Source: CAD feature listing. Evaluate the final solid. Frame: model axes, mm. A direction names the side the tool comes from. Round coordinates to 2 decimals unless told otherwise and drop trailing zeros. Order: outer loops, then holes, each group sorted by start corner. A loop starts at its lowest first (then second) coordinate and runs counter-clockwise, first axis right, second up. Notation, with made-up numbers: (-28.5, 2.5) -> (16.5, 2.5) arc R7 ccw to (16.5, 9.5) -> close; hole circle Ø6 at (78.5, 54.25). An arc over 180 degrees is marked (long way). Answer as CSV lines item,"result". Start each with the question number.
(1) Section query B-B (y = -12.5). Output: boundary loops of the cut face in (x, z).
(2) Set-up query: faces 5 (the flat face through (52, -12, 10)), 6 (the flat face through (75, -12, 2)), 7 (the flat face through (-52, -12, 10)). Return all of +Z, -Z, +X, -X, +Y, -Y with unobstructed straight access to the full face (end or side cutting, diameter ignored); none if empty.
(3) Contact query for flat-ended pins moving along their axis: P1, Ø12, axis at y = -13.5, z = 44, coming from the -X side; P2, Ø2, axis at y = -6.5, z = 26.5, coming from the -X side; P3, Ø10, axis at x = 52, y = -10, coming from the +Z side; P4, Ø13.5, axis at x = 60, y = -12.5, coming from the +Z side. Output: stop coordinate, or through.
(4) Pull-direction query (Y, two-part tool) for faces 1 (the flat face through (-1, -25, 22)), 2 (the cylindrical face through (52.507, -12.17, 5.07)), 3 (the cylindrical face through (-67.493, -12.17, 5.07)), 4 (the flat face through (-1, -12, 0)); classes: +Y half, -Y half, draft (parallel to the pull), parting line (faces both ways), or undercut.
(5) Line query: line 1 along X through (y, z) = (-9.75, 8); line 2 along Y through (x, z) = (60, 6); line 3 along Z through (x, y) = (-57.5, -2.5). Output: solid intervals per line, ascending. Write a range as from..to.
(6) Section query A-A (x = 60). Output: boundary loops of the cut face in (y, z), plus the area to 3 significant figures.
(7) Section query D-D (x = -54.5). Output: boundary loops of the cut face in (y, z), plus the area to 3 significant figures.
(8) Section query C-C (y = -22.25). Output: boundary loops of the cut face in (x, z).
```python
from build123d import *

# Parameters (mm, degrees)
F1_DEPTH = 25
F2_R     = 7.5
F3_DEPTH = 10.001


with BuildPart() as f1:
    # F0 (on Front) → F1 (new body)
    with BuildSketch(Plane.XZ):
        with BuildLine():
            Line((-45, 10), (-45, 0))
            Line((-45, 0), (45, 0))
            Line((45, 0), (45, 10))
            ThreePointArc((45, 10), (31.819805, 41.819805), (0, 55))
            ThreePointArc((0, 55), (-31.819805, 41.819805), (-45, 10))
        make_face()
        with BuildLine():
            Line((-75, 5), (-75, 0))
            Line((-75, 0), (-45, 0))
            Line((-45, 0), (-45, 10))
            Line((-45, 10), (-70, 10))
            ThreePointArc((-70, 10), (-73.535534, 8.535534), (-75, 5))
        make_face()
        with BuildLine():
            Line((45, 10), (45, 0))
            Line((45, 0), (75, 0))
            Line((75, 0), (75, 5))
            ThreePointArc((75, 5), (73.535534, 8.535534), (70, 10))
            Line((70, 10), (45, 10))
        make_face()
    extrude(amount=F1_DEPTH)

    # F2 (on face) → F3 (cut, through all)
    with BuildSketch(Plane.XY.offset(10)):
        with Locations((-60, -12.5)):
            Circle(F2_R)
        with Locations((60, -12.5)):
            Circle(F2_R)
    extrude(amount=-F3_DEPTH, mode=Mode.SUBTRACT)


solid = f1.part
```
Answer block:
1,outline,"(-75, 0) -> (-67.5, 0) -> (-67.5, 10) -> (-70, 10) arc R5 ccw to (-75, 5) -> close; (-52.5, 0) -> (52.5, 0) -> (52.5, 10) -> (45, 10) arc R45 ccw to (0, 55) arc R45 ccw to (-45, 10) -> (-52.5, 10) -> close; (67.5, 0) -> (75, 0) -> (75, 5) arc R5 ccw to (70, 10) -> (67.5, 10) -> close"
2,face 5,"+Z, +X, +Y, -Y"
2,face 6,"+Z, -Z, +X, +Y, -Y"
2,face 7,"+Z, -X, +Y, -Y"
3,P1,"x = -35.23"
3,P2,"x = -42.25"
3,P3,"z = 10"
3,P4,"through"
4,face 1,"-Y half"
4,face 2,"undercut"
4,face 3,"undercut"
4,face 4,"draft"
5,line 1,"-74..-66.98, -53.02..53.02, 66.98..74"
5,line 2,"-25..-20, -5..0"
5,line 3,"0..10"
6,outline,"(-25, 0) -> (-20, 0) -> (-20, 10) -> (-25, 10) -> close; (-5, 0) -> (0, 0) -> (0, 10) -> (-5, 10) -> close"
6,area,"100 mm2"
7,outline,"(-25, 0) -> (-17.6, 0) -> (-17.6, 10) -> (-25, 10) -> close; (-7.4, 0) -> (0, 0) -> (0, 10) -> (-7.4, 10) -> close"
7,area,"148 mm2"
8,outline,"(-75, 0) -> (75, 0) -> (75, 5) arc R5 ccw to (70, 10) -> (45, 10) arc R45 ccw to (0, 55) arc R45 ccw to (-45, 10) -> (-70, 10) arc R5 ccw to (-75, 5) -> close"
